Solid Edge part; units mm, degrees
sketch "Sketch1" plane through (0, 0, 0) normal (1, 0, 0) x (0, 1, 0)
  circle A0 centre (0, 0) radius 14.78
extrude "Protrusion1" add sketch "Sketch1" against normal blind 25.4
sketch "Sketch2" plane through (0, 0, 0) normal (1, 0, 0) x (0, 1, 0)
  circle A0 centre (0, 0) radius 5
extrude "Cutout1" cut sketch "Sketch2" against normal up to next
sketch "Sketch3" plane through (0, 0, 0) normal (1, 0, 0) x (0, 1, 0)
  line L0 (2.424, 14.5799) -> (1.525, 12.11)
  line L1 (1.525, 12.11) -> (-1.525, 12.11)
  line L2 (-1.525, 12.11) -> (-2.424, 14.5799)
  arc A0 (2.424, 14.5799) -> (-2.424, 14.5799) centre (0, 0) ccw
extrude "Cutout2" cut sketch "Sketch3" against normal blind 14000
pattern_circular "Pattern1" count 10 over 360 about axis through (0, 0, 0) along (1, 0, 0) of "Cutout2"
properties material "Steel"
Could you check a few things on this model? Use its own coordinates, in mm. A direction names the side the tool comes from. Give positions to 0.01 mm unless a question says otherwise; leave off trailing zeros. Order: outer loops, then holes, each group sorted by start corner. A loop starts at its lowest first (then second) coordinate and runs counter-clockwise, first axis right, second up.
1. Suppose I cut it at B-B (y = 0). List the corners of the cut face in (x, z) for me.
2. Suppose I cut it at A-A (z = 0). List the corners of the cut face in (x, y) for me, plus the area to 3 significant figures.
3. Will these pins go through, and if not, where does the flat tip stop? P1, Ø3, axis at x = -11.5, y = 11.5, coming from the +Z side; P2, Ø12, axis at x = -22.5, z = -9, coming from the -Y side; P3, Ø2, axis at x = -9, y = -10.5, coming from the -Z side; P4, Ø8, axis at y = 0, z = 0, coming from the -X side.
4. For faces 1 (the flat face through (-12.52, -7.1, 9.81)), 2 (the flat face through (-12.52, 6.25, -11.97)), 3 (the flat face through (-12.52, 9.46, 9.65)), 4 (the flat face through (-12.522, -12.067, -5.99)), 5 (the flat face through (-12.52, -9.46, -9.65)), which set-ups out of +Z, -Z, +X, -X, +Y, -Y let a thin tool reach every point of the face, with its end or its side?
5. We'd pull the mould along Z, two halves only. Please class faces 6 (the flat face through (-12.52, -9.43, 9.63)), 7 (the flat face through (-12.522, -12.096, 6.013)), 8 (the cylindrical face through (-12.522, -4.597, -14.047)): pulls with the +Z half, pulls with the -Z half, needs draft (parallel to the pull), parting line crosses it, or undercut.
6. I need wall thicknesses on L1, parallel to Z at x = -15.75, y = 0; L2, parallel to Z at x = -8.75, y = -12.5; L3, parallel to Y at x = -5.75, z = 9.5. Which ranges of each line are inside material? Lowest first, please.
7. Suppose I cut it at C-C (z = 8). List the corners of the cut face in (x, y) for me.
Solved:
1. outline: (-25.4, -12.11) - (0, -12.11) - (0, -5) - (-25.4, -5) - close; (-25.4, 5) - (0, 5) - (0, 12.11) - (-25.4, 12.11) - close
2. outline: (-25.4, -14.78) - (0, -14.78) - (0, -5) - (-25.4, -5) - close; (-25.4, 5) - (0, 5) - (0, 14.78) - (-25.4, 14.78) - close
2. area: 497 mm2
3. P1: stops at z = 10.37
3. P2: stops at y = -13.12
3. P3: stops at z = -10.37
3. P4: passes through
4. face 1: +X, -X
4. face 2: +X, -X, +Y
4. face 3: +Z, +X, -X
4. face 4: +X, -X, -Y
4. face 5: -Z, +X, -X
5. face 6: pulls with the +Z half
5. face 7: undercut
5. face 8: pulls with the -Z half
6. L1: z = -12.11 to -5, 5 to 12.11
6. L2: z = -7.89 to -6.33, -2.27 to 2.27, 6.33 to 7.89
6. L3: y = -11.32 to -9.24, -7.53 to 7.53, 9.24 to 11.32
7. outline: (-25.4, -12.43) - (0, -12.43) - (0, 12.43) - (-25.4, 12.43) - close
